Verification items for the finished model (mm, model axes). Face numbers are marked on the shaded views. A direction names the side the tool comes from. Coordinates: 2 decimals unless noted, no trailing zeros. Order: outer loops, then holes, each group sorted by start corner. A loop starts at its lowest first (then second) coordinate and runs counter-clockwise, first axis right, second up. Notation, with made-up numbers: (44.5, 14.25) -> (78.5, 14.25) arc R17 cw to (78.5, 22.25) -> close; hole circle Ø2 at (2, -16). An arc over 180 degrees is marked (long way). Write each question's results on one line, items separated by ' | '. Start each with the question number.
(1) Set-up check for the marked faces 4, 5 and 6: record each of +Z, -Z, +X, -X, +Y, -Y from which the full face is reachable in a straight line by a thin tool's end or side.
(2) Thickness scan on probe 1 along Y at (x, z) = (0, 3.25) (3 decimals); probe 2 along X at (y, z) = (4, 9). Record the ranges inside material, lowest first. Write a range as [from, to].
(3) Go/stop test with flat-tipped pins: pin 1 (2.5 mm diameter, centred on x = 1, y = 0.5, fed in from -Z); pin 2 (1.4 mm diameter, centred on x = 4, y = -4.5, fed in from -Z); pin 3 (1.5 mm diameter, centred on x = 0, y = -6, fed in from +Z). Record where each tip stops, or that it passes through.
(4) Cross-section at B-B on x = 0. Enter the section's corners in (y, z) (3 decimals), and give its area (3 significant figures).
(5) Cross-section at C-C on z = 9. Enter the section's corners in (x, y).
(6) Draft check along X on the marked faces 1, 2 and 3. Enter one of: +X half, -X half, draft (parallel to the pull), parting line (faces both ways), or undercut.
(7) Cross-section at D-D on y = 4. Enter the section's corners in (x, z).
(8) Cross-section at A-A on z = 5.5. Enter the section's corners in (x, y) (3 decimals).
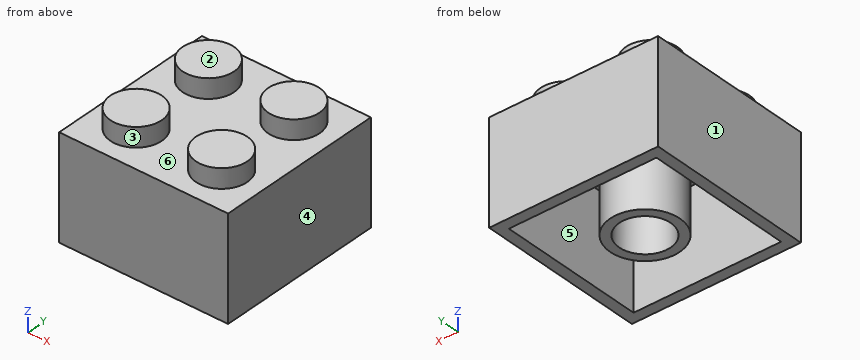
```python
from build123d import *

# Parameters (mm, degrees)
F0_W     = 15.8
F0_H     = 15.8
F1_DEPTH = 9.6
F2_R     = 2.4
F3_DEPTH = 1.8
F4_T     = -1
F5_R     = 3.255
F5_R_2   = 2.4
F6_DEPTH = 8.6


with BuildPart() as f1:
    # F0 (on Top) → F1 (new body)
    with BuildSketch(Plane.XY):
        Rectangle(F0_W, F0_H)
    extrude(amount=F1_DEPTH)

    # F2 (on face) → F3 (join)
    with BuildSketch(Plane.XY.offset(9.6)):
        with Locations((-4, 4)):
            Circle(F2_R)
        with Locations((4, 4)):
            Circle(F2_R)
        with Locations((4, -4)):
            Circle(F2_R)
        with Locations((-4, -4)):
            Circle(F2_R)
    extrude(amount=F3_DEPTH)

    # F4
    f4_openings = [f1.faces().sort_by_distance(p)[0] for p in [
        (0, 0, 0),
    ]]
    offset(amount=F4_T, openings=f4_openings, kind=Kind.INTERSECTION)

    # F5 (on face) → F6 (join, through all)
    with BuildSketch(Plane(origin=(0, 0, 8.6), x_dir=(1, 0, 0), z_dir=(0, 0, -1))):
        Circle(F5_R)
        Circle(F5_R_2, mode=Mode.SUBTRACT)
    extrude(amount=F6_DEPTH)


solid = f1.part
```
Results are:
1) face 4: +Z, -Z, +X, +Y, -Y | face 5: -Z | face 6: +Z
2) probe 1: y = [-7.9, -6.9], [-3.255, -2.4], [2.4, 3.255], [6.9, 7.9] | probe 2: x = [-7.9, -5.4], [-2.6, 2.6], [5.4, 7.9]
3) pin 1: stops at z = 8.6 | pin 2: stops at z = 10.4 | pin 3: stops at z = 9.6
4) outline: (-7.9, 0) -> (-6.9, 0) -> (-6.9, 8.6) -> (-3.255, 8.6) -> (-3.255, 0) -> (-2.4, 0) -> (-2.4, 8.6) -> (2.4, 8.6) -> (2.4, 0) -> (3.255, 0) -> (3.255, 8.6) -> (6.9, 8.6) -> (6.9, 0) -> (7.9, 0) -> (7.9, 9.6) -> (-7.9, 9.6) -> close | area: 47.7 mm2
5) outline: (-7.9, -7.9) -> (7.9, -7.9) -> (7.9, 7.9) -> (-7.9, 7.9) -> close; hole circle Ø2.8 at (-4, -4); hole circle Ø2.8 at (-4, 4); hole circle Ø2.8 at (4, -4); hole circle Ø2.8 at (4, 4)
6) face 1: -X half | face 2: draft | face 3: undercut
7) outline: (-7.9, 0) -> (-6.9, 0) -> (-6.9, 8.6) -> (-5.4, 8.6) -> (-5.4, 10.4) -> (-2.6, 10.4) -> (-2.6, 8.6) -> (2.6, 8.6) -> (2.6, 10.4) -> (5.4, 10.4) -> (5.4, 8.6) -> (6.9, 8.6) -> (6.9, 0) -> (7.9, 0) -> (7.9, 9.6) -> (6.4, 9.6) -> (6.4, 11.4) -> (1.6, 11.4) -> (1.6, 9.6) -> (-1.6, 9.6) -> (-1.6, 11.4) -> (-6.4, 11.4) -> (-6.4, 9.6) -> (-7.9, 9.6) -> close
8) outline: (-7.9, -7.9) -> (7.9, -7.9) -> (7.9, 7.9) -> (-7.9, 7.9) -> close; circle Ø6.51 at (0, 0); hole (-6.9, -6.9) -> (6.9, -6.9) -> (6.9, 6.9) -> (-6.9, 6.9) -> close; hole circle Ø4.8 at (0, 0)
